Geometry: final body of the model. Coordinates: model frame, mm. A direction names the side the tool comes from. Give positions to 0.01 mm unless a question says otherwise; leave off trailing zeros. Write each loop counter-clockwise with the first axis right and the second up, starting at its lowest first coordinate (ties: lowest second). Pieces come first, ordered by that corner, then holes.
```python
from build123d import *

# Parameters (mm, degrees)
SKETCH1_R           = 13.7
BOSS_EXTRUDE1_DEPTH = 1
CHAMFER2_SIZE       = 1
SKETCH4_R           = 3
BOSS_EXTRUDE2_DEPTH = 97.8
FILLET1_R           = 12
SKETCH5_W           = 0.49999999999999956
SKETCH5_H           = 1


# Some blends are built 0.0001 mm under size
with BuildPart() as part:
    # Sketch1 → Boss-Extrude1 (new body)
    with BuildSketch(Plane(origin=(0, 0, 0), x_dir=(1, 0, 0), z_dir=(0, 1, 0))):
        with Locations(Location((0, 0, 0), (0, 0, 270))):
            Circle(SKETCH1_R)
    extrude(amount=BOSS_EXTRUDE1_DEPTH)

    # Chamfer2
    chamfer2_edges = [part.edges().sort_by_distance(p)[0] for p in [
        (4.19e-15, 1, -13.7),
    ]]
    chamfer(chamfer2_edges, length=CHAMFER2_SIZE - 0.0001)  # a hair under: the kernel refuses the full size

    # Sketch4 → Boss-Extrude2 (add)
    with BuildSketch(Plane(origin=(0, 1, 0), x_dir=(1, 0, 0), z_dir=(0, 1, 0))):
        with Locations(Location((0, 0, 0), (0, 0, 270))):
            Circle(SKETCH4_R)
    extrude(amount=BOSS_EXTRUDE2_DEPTH)

    # Fillet1
    # the kernel refuses this fillet: 12 mm, written as the material it adds along each edge
    with BuildSketch(Plane(origin=(0, 1, 0), x_dir=(-1.8e-16, 0, 1), z_dir=(-1, 0, -1.8e-16))) as fillet1_piece_1:
        with BuildLine():
            CenterArc((15, 11.777540489856218), FILLET1_R, 180, 78.95042152448133)
            Line((3, 11.777540489856218), (2.76, 11.777540489856218))
            Line((2.76, 11.777540489856218), (2.76, 0))
            Line((2.76, 0), (3, -0.24))
            ThreePointArc((3, -0.24), (7.850050000000809, -0.24), (12.65410200000165, -0.23555080978867193))
            Line((12.65410200000165, -0.23555080978867193), (12.700100000001617, 8.2867e-12))
        make_face()
    revolve(axis=Axis((0, 1, 0), (0, 1, 0)))

    # Sketch5 → Cut-Revolve1 (revolve, cut)
    with BuildSketch(Plane.XY, mode=Mode.PRIVATE) as cut_revolve1_sk:
        with Locations((-2.75, 93.30000000000001)):
            Rectangle(SKETCH5_W, SKETCH5_H)
        with Locations((-2.75, 91.3)):
            Rectangle(SKETCH5_W, SKETCH5_H)
        Polygon((-2.500000000000001, 89.8), (-2.5000000000000004, 88.79999999999998), (-3.0000000000000004, 88.79999999999998), (-3.0000000000000004, 89.8), align=None)
    revolve(cut_revolve1_sk.sketch.rotate(Axis((0, 98.8, 0), (0, -1, 0)), 270), axis=Axis((0, 98.8, 0), (0, -1, 0)), mode=Mode.SUBTRACT)


solid = part.part
```
Item 1: Reachability of faces 1 (the face through (0.9, 92.29, 2.86)), 2 (the face through (-2, 92.8, -2)) from +Z, -Z, +X, -X, +Y, -Y: full face, straight path, thin tool, end or side. Return the list, or none.
Found:
face 1: +Y
face 2: none
Item 2: Line query: L1, parallel to Y at x = 6, z = -8.5; L2, parallel to Y at x = -8, z = -1; L3, parallel to X at y = 79, z = -1. Output: solid intervals per line, ascending.
Found:
L1: y = 0 to 1.69
L2: y = 0 to 2.99
L3: x = -2.83 to 2.83
Item 3: Pull-direction query (Y, two-part tool) for faces 3 (the face through (0, 98.8, 0)), 4 (the face through (0.9, 96.26, 2.86)), 5 (the face through (0, 0, 0)), 6 (the face through (-2, 93.8, -2)); classes: +Y half, -Y half, draft (parallel to the pull), parting line (faces both ways), or undercut.
Found:
face 3: +Y half
face 4: draft
face 5: -Y half
face 6: undercut
Item 4: Section D-D, the plane y = 11.5. Return the cut outline in (x, z).
Found:
outline: circle Ø6.14 at (0, 0)
Item 5: Section C-C, the plane y = 82.5. Return the cut outline in (x, z).
Found:
outline: circle Ø6 at (0, 0)
Item 6: Pin query (flat end, axial travel): pin 1 Ø8 at (y, z) = (43, -2.5) entering from +X; pin 2 Ø6 at (x, y) = (-2, 71) entering from +Z; pin 3 Ø5 at (y, z) = (12, -1.5) entering from -X. Return the tip coordinate at first contact, or that it passes through.
Found:
pin 1: stops at x = 3
pin 2: stops at z = 3
pin 3: stops at x = -3.36
